```python
from build123d import *

# Parameters (mm, degrees)
SKETCH_1_W               = 80
SKETCH_1_H               = 30
EXTRUDE_1_DEPTH          = 2
SKETCH_2_R               = 2.5
EXTRUDE_2_DEPTH          = 5
SKETCH_3_R               = 1.25
CUT_EXTRUDE_1_DEPTH      = 1
CUT_EXTRUDE_1_DEPTH_BACK = 8
SKETCH_4_R               = 2
CUT_EXTRUDE_2_DEPTH      = 6
CUT_EXTRUDE_2_DEPTH_BACK = 3
FILLET_1_R               = 2
FILLET_2_R               = 2
FILLET_3_R               = 2
FILLET_4_R               = 2


with BuildPart() as part:
    # Эскиз1 → Бобышка-Вытянуть1 (new body)
    with BuildSketch(Plane(origin=(0, 0, 0), x_dir=(1, 0, 0), z_dir=(0, 1, 0))):
        with Locations((40, -15)):
            Rectangle(SKETCH_1_W, SKETCH_1_H)
    extrude(amount=EXTRUDE_1_DEPTH)

    # Эскиз2 → Бобышка-Вытянуть2 (add)
    with BuildSketch(Plane(origin=(0, 2, 0), x_dir=(1, 0, 0), z_dir=(0, 1, 0))):
        with Locations((12, -5.5)):
            Circle(SKETCH_2_R)
        with Locations((12, -24.5)):
            Circle(SKETCH_2_R)
        with Locations((68, -5.5)):
            Circle(SKETCH_2_R)
        with Locations((68, -24.5)):
            Circle(SKETCH_2_R)
    extrude(amount=EXTRUDE_2_DEPTH)

    # Эскиз3 → Вырез-Вытянуть1 (cut, two sides)
    with BuildSketch(Plane(origin=(0, 7, 0), x_dir=(1, 0, 0), z_dir=(0, 1, 0))) as cut_extrude_1_sk:
        with Locations((12, -5.5)):
            Circle(SKETCH_3_R)
        with Locations((12, -24.5)):
            Circle(SKETCH_3_R)
        with Locations((68, -5.5)):
            Circle(SKETCH_3_R)
        with Locations((68, -24.5)):
            Circle(SKETCH_3_R)
    extrude(amount=CUT_EXTRUDE_1_DEPTH, mode=Mode.SUBTRACT)
    extrude(cut_extrude_1_sk.sketch, amount=-CUT_EXTRUDE_1_DEPTH_BACK, mode=Mode.SUBTRACT)

    # Эскиз4 → Вырез-Вытянуть2 (cut, two sides)
    with BuildSketch(Plane(origin=(0, 2, 0), x_dir=(1, 0, 0), z_dir=(0, 1, 0))) as cut_extrude_2_sk:
        with Locations((4.5, -5)):
            Circle(SKETCH_4_R)
        with Locations((75.5, -15)):
            Circle(SKETCH_4_R)
    extrude(amount=CUT_EXTRUDE_2_DEPTH, mode=Mode.SUBTRACT)
    extrude(cut_extrude_2_sk.sketch, amount=-CUT_EXTRUDE_2_DEPTH_BACK, mode=Mode.SUBTRACT)

    # Скругление1
    fillet_1_edges = [part.edges().sort_by_distance(p)[0] for p in [
        (0, 1, 30),
    ]]
    fillet(fillet_1_edges, radius=FILLET_1_R)

    # Скругление2
    fillet_2_edges = [part.edges().sort_by_distance(p)[0] for p in [
        (0, 1, 0),
    ]]
    fillet(fillet_2_edges, radius=FILLET_2_R)

    # Скругление3
    fillet_3_edges = [part.edges().sort_by_distance(p)[0] for p in [
        (80, 1, 0),
    ]]
    fillet(fillet_3_edges, radius=FILLET_3_R)

    # Скругление4
    fillet_4_edges = [part.edges().sort_by_distance(p)[0] for p in [
        (80, 1, 30),
    ]]
    fillet(fillet_4_edges, radius=FILLET_4_R)


solid = part.part
```
For this review, take the finished solid that the model builds, in its own axes (mm). A direction names the side the tool comes from. Give positions to 0.01 mm unless a question says otherwise; leave off trailing zeros. Write each loop counter-clockwise with the first axis right and the second up, starting at its lowest first coordinate (ties: lowest second). Pieces come first, ordered by that corner, then holes.
Item 1: Take a section at A-A (z = 24.5). Give the boundary of the cut face in (x, y), and give its area (3 significant figures).
Item 2: Insertion check: P1, Ø4.5, axis at x = 4.5, z = 5, coming from the +Y side. The pin has a flat end and moves straight along its axis. Give the tip position at first contact, or say it passes through.
Item 3: Machinability: for faces 4 (the face through (69, 7, 23)), 5 (the face through (69.34, 4.46, 22.39)), which of the approach directions +Z, -Z, +X, -X, +Y, -Y give a long, thin tool a straight path to every point of the face, cutting with its end or side? Answer none if there is none.
Item 4: Wall thickness on probe 1 along X at (y, z) = (5, 24.5); probe 2 along Z at (x, y) = (68, 3.25); probe 3 along Z at (x, y) = (12, 1.5): over which ranges is each line inside the solid? List them lowest first.
Item 5: The part is to be moulded in two halves that separate along Z. For faces 1 (the face through (69, 7, 4)), 2 (the face through (39, 1, 30)), 3 (the face through (2.9, 1, 6.2)), say which applies: +Z half, -Z half, draft (parallel to the pull), parting line (faces both ways), or undercut.
Item 6: Take a section at B-B (y = 3.5). Give the boundary of the cut face in (x, z), and give its area (3 significant figures).
Item 7: Take a section at D-D (x = 75.5). Give the boundary of the cut face in (y, z).
Item 8: Take a section at C-C (z = 15). Give the boundary of the cut face in (x, y), and give its area (3 significant figures).
Established:
1. outline: (0, 0) - (10.75, 0) - (10.75, 7) - (9.5, 7) - (9.5, 2) - (0, 2) - close; (13.25, 0) - (66.75, 0) - (66.75, 7) - (65.5, 7) - (65.5, 2) - (14.5, 2) - (14.5, 7) - (13.25, 7) - close; (69.25, 0) - (80, 0) - (80, 2) - (70.5, 2) - (70.5, 7) - (69.25, 7) - close
1. area: 175 mm2
2. P1: stops at y = 2
3. face 4: +Z, -Z, +X, -X, +Y
3. face 5: +Y
4. probe 1: x = 9.5 to 10.75, 13.25 to 14.5, 65.5 to 66.75, 69.25 to 70.5
4. probe 2: z = 3 to 4.25, 6.75 to 8, 22 to 23.25, 25.75 to 27
4. probe 3: z = 0 to 4.25, 6.75 to 23.25, 25.75 to 30
5. face 1: draft
5. face 2: +Z half
5. face 3: undercut
6. outline: circle Ø5 at (12, 5.5); circle Ø5 at (12, 24.5); circle Ø5 at (68, 5.5); circle Ø5 at (68, 24.5); hole circle Ø2.5 at (12, 5.5); hole circle Ø2.5 at (12, 24.5); hole circle Ø2.5 at (68, 5.5); hole circle Ø2.5 at (68, 24.5)
6. area: 58.9 mm2
7. outline: (0, 0) - (2, 0) - (2, 13) - (0, 13) - close; (0, 17) - (2, 17) - (2, 30) - (0, 30) - close
8. outline: (0, 0) - (73.5, 0) - (73.5, 2) - (0, 2) - close; (77.5, 0) - (80, 0) - (80, 2) - (77.5, 2) - close
8. area: 152 mm2
